from build123d import *

# Parameters (mm, degrees)
SKETCH_1_W             = 3.5
SKETCH_1_H             = 13
EXTRUDE_1_DEPTH        = 26
SKETCH_3_R             = 2.2
EXTRUDE_3_DEPTH        = 6.5
HOLE_WIZARD_M2_1_D     = 1.6
HOLE_WIZARD_M2_1_DEPTH = 6
HOLE_WIZARD_M2_1_TIP   = 0.480688495
SKETCH_6_W             = 5.854472115
SKETCH_6_H             = 12.222775643
EXTRUDE_4_DEPTH        = 3
F_2_0MM_1_D            = 2.3
F_2_0MM_1_DEPTH        = 4.15
F_2_0MM_1_TIP          = 0.690989712
FILLET_2_R             = 1
FILLET_3_R             = 1
FILLET_4_R             = 1
FILLET_5_R             = 1
FILLET_6_R             = 1
SKETCH_9_W             = 7.566336663
SKETCH_9_H             = 6.401025682
EXTRUDE_5_DEPTH        = 3.5
SKETCH_10_R            = 1.85
EXTRUDE_6_DEPTH        = 3.7
FILLET_7_R             = 1


with BuildPart() as part:
    # 草图1 → 凸台-拉伸1 (new body)
    with BuildSketch(Plane.XY):
        with Locations((0.621335505, 0.911868233)):
            Rectangle(SKETCH_1_W, SKETCH_1_H)
    extrude(amount=EXTRUDE_1_DEPTH)

    # 草图3 → 凸台-拉伸3 (add)
    with BuildSketch(Plane.ZY.offset(1.128664495)):
        with Locations(Location((6.16, 1.411868233, 0), (0, 0, 90))):
            Circle(SKETCH_3_R)
        with Locations(Location((18.16, 1.411868233, 0), (0, 0, 90))):
            Circle(SKETCH_3_R)
    extrude(amount=EXTRUDE_3_DEPTH)

    # M2 螺纹孔1
    with Locations(Plane.XZ.offset(5.588131767)):
        with Locations((0.621335505, 9), (0.621335505, 18)):
            Hole(HOLE_WIZARD_M2_1_D / 2, depth=HOLE_WIZARD_M2_1_DEPTH)
            with Locations((0, 0, -(HOLE_WIZARD_M2_1_DEPTH + HOLE_WIZARD_M2_1_TIP / 2))):  # 118° drill point
                Cone(0, HOLE_WIZARD_M2_1_D / 2, HOLE_WIZARD_M2_1_TIP, mode=Mode.SUBTRACT)

    # 草图6 → 凸台-拉伸4 (add)
    with BuildSketch(Plane.XZ.offset(5.588131767)):
        with Locations((5.298571563, 14.336084675)):
            Rectangle(SKETCH_6_W, SKETCH_6_H)
    extrude(amount=-EXTRUDE_4_DEPTH)

    # Ø2.0mm 暗销孔1
    with Locations(Plane.XZ.offset(5.588131767)):
        with Locations((4.621335505, 13.5)):
            Hole(F_2_0MM_1_D / 2, depth=F_2_0MM_1_DEPTH)
            with Locations((0, 0, -(F_2_0MM_1_DEPTH + F_2_0MM_1_TIP / 2))):  # 118° drill point
                Cone(0, F_2_0MM_1_D / 2, F_2_0MM_1_TIP, mode=Mode.SUBTRACT)

    # 圆角2
    fillet_2_edges = [part.edges().sort_by_distance(p)[0] for p in [
        (2.371335505, -2.588131767, 14.336084675),
    ]]
    fillet(fillet_2_edges, radius=FILLET_2_R)

    # 圆角3
    fillet_3_edges = [part.edges().sort_by_distance(p)[0] for p in [
        (2.371335505, -3.588131767, 20.447472496),
    ]]
    fillet(fillet_3_edges, radius=FILLET_3_R)

    # 圆角4
    fillet_4_edges = [part.edges().sort_by_distance(p)[0] for p in [
        (2.371335505, -3.588131767, 8.224696853),
    ]]
    fillet(fillet_4_edges, radius=FILLET_4_R)

    # 圆角5
    fillet_5_edges = [part.edges().sort_by_distance(p)[0] for p in [
        (8.22580762, -4.088131767, 8.224696853),
    ]]
    fillet(fillet_5_edges, radius=FILLET_5_R)

    # 圆角6
    fillet_6_edges = [part.edges().sort_by_distance(p)[0] for p in [
        (8.22580762, -4.088131767, 20.447472496),
    ]]
    fillet(fillet_6_edges, radius=FILLET_6_R)

    # 草图9 → 凸台-拉伸5 (add)
    with BuildSketch(Plane.ZY.offset(1.128664495)):
        with Locations((22.216831668, 10.612381074)):
            Rectangle(SKETCH_9_W, SKETCH_9_H)
    extrude(amount=-EXTRUDE_5_DEPTH)

    # 草图10 → 凸台-拉伸6 (add)
    with BuildSketch(Plane.ZY.offset(1.128664495)):
        with Locations(Location((20.85, 11.722893915, 0), (0, 0, 90))):
            Circle(SKETCH_10_R)
    extrude(amount=EXTRUDE_6_DEPTH)

    # 圆角7
    fillet_7_edges = [part.edges().sort_by_distance(p)[0] for p in [
        (0.621335505, 7.411868233, 18.433663337),
    ]]
    fillet(fillet_7_edges, radius=FILLET_7_R)


solid = part.part
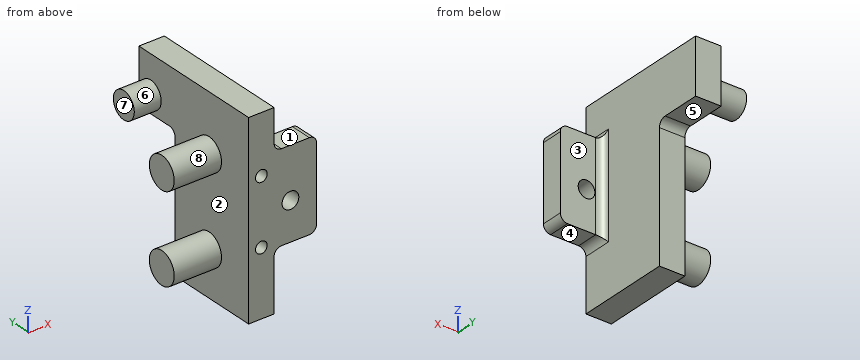
CAD build for the part. Positions are in the model's coordinates, mm. Face numbers are marked on the shaded views. A direction names the side the tool comes from. Coordinates: 2 decimals unless noted, no trailing zeros. Write each loop counter-clockwise with the first axis right and the second up, starting at its lowest first coordinate (ties: lowest second). Pieces come first, ordered by that corner, then holes. Notation, with made-up numbers: M -22.75,2.5 L -18.75,2.5 A17 ccw -18.75,15.5 Z; hole C 8,-31.75 d9. An arc over 180 degrees is marked long. Answer as a JSON object with one key per item and string values. Group by question number.
1) Pin check, flat tips, straight feed: pin 1 Ø8 at (x, z) = (5.5, 7.5) entering from -Y; pin 2 Ø1 at (x, z) = (0.5, 8.5) entering from +Y; pin 3 Ø0.9 at (x, y) = (6, -4) entering from +Z; pin 4 Ø6 at (y, z) = (6.5, 10.5) entering from -X. Stop position of each tip, or through.
2) Saw through at A-A (x = 4.5). Write the cut outline in (y, z).
3) Mould opens along Z. For the marked faces 6, 7 and 8 say: +Z half, -Z half, draft (parallel to the pull), parting line (faces both ways), or undercut.
4) Saw through at D-D (z = 10.75). Write the cut outline in (x, y), plus the area to 3 significant figures.
5) Saw through at B-B (z = 14). Write the cut outline in (x, y), plus the area to 3 significant figures.
6) Saw through at C-C (x = -2.25). Write the cut outline in (y, z).
7) Tool access for the marked faces 1, 2, 3, 4 and 5: list every direction of +Z, -Z, +X, -X, +Y, -Y with a clear straight run to the whole face (end or side of a thin tool).
8) Wall check: line 1 (X direction, y = -2.75, z = 18); line 2 (X direction, y = 5, z = 14.75); line 3 (Y direction, x = -3.75, z = 19.25). Give the ranges that are in metal, low to high. Write a range as from..to.
Values follow:
{
 "1": {"pin 1": "stops at y = -5.59", "pin 2": "stops at y = 7.41", "pin 3": "stops at z = 20.45", "pin 4": "stops at x = -1.13"},
 "2": {"outline": "M -5.59,8.22 L -2.59,8.22 L -2.59,12.36 L -5.59,12.36 Z; M -5.59,14.64 L -2.59,14.64 L -2.59,20.45 L -5.59,20.45 Z"},
 "3": {"face 6": "parting line", "face 7": "draft", "face 8": "undercut"},
 "4": {"outline": "M -1.13,-5.59 L 8.23,-5.59 L 8.23,-2.59 L 3.37,-2.59 A1 cw 2.37,-1.59 L 2.37,7.41 L -1.13,7.41 Z", "area": "63.3 mm2"},
 "5": {"outline": "M -1.13,-5.59 L 3.59,-5.59 L 3.59,-2.59 L 3.37,-2.59 A1 cw 2.37,-1.59 L 2.37,7.41 L -1.13,7.41 Z; M 5.66,-5.59 L 8.23,-5.59 L 8.23,-2.59 L 5.66,-2.59 Z", "area": "57.1 mm2"},
 "6": {"outline": "C 1.41,6.16 d4.4; C 1.41,18.16 d4.4; C 11.72,20.85 d3.7"},
 "7": {"face 1": "+Z, +X, +Y, -Y", "face 2": "-X", "face 3": "+Z, -Z, +X, +Y", "face 4": "-Z, +X, +Y, -Y", "face 5": "-Z, +X, -X, +Y"},
 "8": {"line 1": "x = -1.13..-0.18, 1.42..8.23", "line 2": "x = -1.13..2.37", "line 3": "y = -0.5..3.32, 10.79..12.65"}
}
